Autodesk Inventor part; units mm, degrees
ref_plane "YZ Plane" through (0, 0, 0) normal (1, 0, 0) x (0, 1, 0)
ref_plane "XZ Plane" through (0, 0, 0) normal (0, 1, 0) x (-1, 0, 0)
ref_plane "XY Plane" through (0, 0, 0) normal (0, 0, 1) x (1, 0, 0)
sketch "Sketch1" plane through (0, 0, 0) normal (0, 0, 1) x (1, 0, 0)
  circle A0 centre (0, 0) radius 31.206
  dimension "d0" = 62.412
extrude "Extrusion1" add sketch "Sketch1" along normal blind 3.175
sketch "Sketch2" plane through (0, 0, 3.175) normal (0, 0, 1) x (1, 0, 0)
  circle A0 centre (0, 0) radius 31.206
  circle A1 centre (0, 0) radius 29.5
  dimension "d3" = 59
sketch "Sketch3" plane through (0, 0, 3.175) normal (0, 0, 1) x (1, 0, 0)
  line L0 (0, 0) -> (-20, 0)
  line L1 (-20, 0) -> (-20, 18)
  line L2 (-20, 18) -> (-23.175, 18)
  line L3 (-23.175, 18) -> (-23.175, -18)
  line L4 (-23.175, -18) -> (-20, -18)
  line L5 (-20, -18) -> (-20, 18)
  dimension "d4" = 20
  dimension "d5" = 18
  dimension "d6" = 3.175
  dimension "d7" = 36
extrude "Extrusion2" add sketch "Sketch3" along normal blind 52
sketch "Sketch4" plane through (-20, -18, 3.175) normal (1, 0, 0) x (0, 0, -1)
  line L0 (0, 49.206) -> (0, -13.206)
  line L1 (-52, 36) -> (-52, 0)
  line L2 (-27, 18) -> (-3, 18)
  line L3 (-3, 18) -> (-51, 18)
  line L4 (-27, 18) -> (-41, 18)
  line L5 (-41, 18) -> (-13, 18)
  circle A0 centre (-41, 18) radius 10
  circle A1 centre (-13, 18) radius 10
  line L6 (-13, 18) -> (-41, 18)
  line L7 (-41, 18) -> (-41, 24.5)
  line L8 (-41, 24.5) -> (-13, 24.5)
  line L9 (-13, 24.5) -> (-13, 18)
  line L10 (-41, 24.5) -> (-13, 24.5)
  line L11 (-13, 24.5) -> (-13, 11.5)
  line L12 (-13, 11.5) -> (-41, 11.5)
  line L13 (-41, 11.5) -> (-41, 24.5)
  point P0 (3.175, 18)
  dimension "d34" = 24
  dimension "d35" = 48
  dimension "d36" = 14
  dimension "d37" = 28
  dimension "d38" = 20
  dimension "d39" = 20
  dimension "d40" = 6.5
  dimension "d41" = 13
extrude "Extrusion3" add sketch "Sketch2" along normal blind 52
sketch "Sketch5" plane through (0, 0, 3.175) normal (0, 0, 1) x (1, 0, 0)
  line L0 (0, 0) -> (0, 23)
  line L1 (0, 23) -> (11.5, 23)
  line L2 (11.5, 23) -> (-11.5, 23)
  line L3 (-11.5, 23) -> (-11.5, -23)
  line L4 (-11.5, -23) -> (11.5, -23)
  line L5 (11.5, -23) -> (11.5, 23)
  circle A0 centre (-11.5, 23) radius 3.5
  circle A1 centre (11.5, 23) radius 3.5
  circle A2 centre (-11.5, -23) radius 3.5
  circle A3 centre (11.5, -23) radius 3.5
  dimension "d16" = 23
  dimension "d17" = 11.5
  dimension "d18" = 23
  dimension "d19" = 46
  dimension "d20" = 7
  dimension "d21" = 7
  dimension "d22" = 7
  dimension "d23" = 7
extrude "Extrusion4" add sketch "Sketch5" along normal blind 52 contours A1 L5 L1 | L1 L5 A1 | A0 L3 L2 | L2 L3 A0 | A3 L4 L5 | L5 L4 A3 | A2 L4 L3 | L3 L4 A2
sketch "Sketch6" plane through (-11.5, 23, 55.175) normal (0, 0, 1) x (1, 0, 0)
  circle A0 centre (0, 0) radius 3.5
  circle A1 centre (23, 0) radius 3.5
  circle A2 centre (23, -46) radius 3.5
  circle A3 centre (0, -46) radius 3.5
  point P0 (11.5, -23)
hole "Hole1" at (-11.5, 23, 55.175) at (11.5, 23, 55.175) at (11.5, -23, 55.175) at (-11.5, -23, 55.175) direction (0, 0, -1) diameter 3.5 depth 3.5
extrude "Extrusion5" cut sketch "Sketch4" along normal blind 52
sketch "Sketch7" plane through (0, 0, 55.175) normal (0, 0, 1) x (1, 0, 0)
  line L0 (-20, 18) -> (-23.175, 18)
  line L1 (-23.175, 18) -> (-23.175, -18)
  line L2 (-20, 18) -> (-23.175, 18)
  line L3 (-23.175, 18) -> (-23.175, -18)
  line L4 (-23.175, -18) -> (-20, -18)
  line L5 (-20, -18) -> (-20, 18)
  point P0 (0, 0)
extrude "Extrusion6" cut sketch "Sketch7" against normal blind 52
properties part number "LidarLiteV3Lid"
Source: CAD feature listing. Evaluate the final solid. Frame: model axes, mm. A direction names the side the tool comes from. Coordinates: 2 decimals unless noted, no trailing zeros. Write each loop counter-clockwise with the first axis right and the second up, starting at its lowest first coordinate (ties: lowest second). Pieces come first, ordered by that corner, then holes. Notation, with made-up numbers: (49.5, -2) -> (69.5, -2) arc R16 cw to (69.5, 9) -> close; hole circle Ø7 at (45, 84). An arc over 180 degrees is marked (long way). Return JSON: item names as keys, results as strings. Group by question number.
1) Contact query for flat-ended pins moving along their axis: P1, Ø1, axis at x = 4, y = -0.5, coming from the +Z side (3 decimals); P2, Ø1, axis at x = -11.5, y = 23, coming from the +Z side (3 decimals); P3, Ø5, axis at y = -15.5, z = 23.5, coming from the +X side. Output: stop coordinate, or through.
2) Mould query, pull axis X, two halves, no side actions, for faces 4 (the face through (-11.58, -21.25, 53.4)), 5 (the face through (30, 6.5, 30)), 6 (the face through (-24.764, 18.988, 27.201)). Classes: +X half, -X half, draft (parallel to the pull), parting line (faces both ways), or undercut.
3) Section query B-B, the plane z = 30.5. Return loops of the section in (x, y), plus the area to 3 significant figures.
4) Ray query, line 1 along X through (y, z) = (-23, 54); line 2 along Y through (x, z) = (13.5, 8); line 3 along Y through (x, z) = (9, 46.5). Return the intervals inside material, ascending.
5) Set-up query: faces 1 (the face through (29.84, 0.34, 6.18)), 2 (the face through (12, -21, 55.175)), 3 (the face through (11.42, -21.25, 53.4)). Return all of +Z, -Z, +X, -X, +Y, -Y with unobstructed straight access to the full face (end or side cutting, diameter ignored); none if empty.
6) Section query C-C, the plane x = 0. Return loops of the section in (y, z) (3 decimals), plus the area to 3 significant figures.
7) Section query A-A, the plane y = 0. Return loops of the section in (x, z) (3 decimals), plus the area to 3 significant figures.
8) Section query D-D, the plane y = 7.5. Return loops of the section in (x, z) (3 decimals).
From the geometry:
{
 "1": {"P1": "z = 3.175", "P2": "z = 51.675", "P3": "x = 28.37"},
 "2": {"face 4": "undercut", "face 5": "draft", "face 6": "parting line"},
 "3": {"outline": "circle Ø7 at (-11.5, -23); circle Ø7 at (-11.5, 23); circle Ø7 at (11.5, -23); circle Ø7 at (11.5, 23); (28.77, -6.5) arc R29.5 cw (long way) to (28.77, 6.5) -> (30.52, 6.5) arc R31.21 ccw (long way) to (30.52, -6.5) -> close", "area": "457 mm²"},
 "4": {"line 1": "-21.09 to -18.47, -15 to -13.25, -9.75 to -8, 8 to 9.75, 13.25 to 15, 18.47 to 21.09", "line 2": "-28.13 to -26.23, -25.87 to -20.13, 20.13 to 25.87, 26.23 to 28.13", "line 3": "-29.88 to -28.09, -25.45 to -20.55, 20.55 to 25.45, 28.09 to 29.88"},
 "5": {"face 1": "+X", "face 2": "+Z, +X, -X, +Y, -Y", "face 3": "+Z"},
 "6": {"outline": "(-31.206, 0) -> (31.206, 0) -> (31.206, 55.175) -> (29.5, 55.175) -> (29.5, 3.175) -> (-29.5, 3.175) -> (-29.5, 55.175) -> (-31.206, 55.175) -> close", "area": "376 mm²"},
 "7": {"outline": "(-31.206, 0) -> (31.206, 0) -> (31.206, 6.175) -> (29.5, 6.175) -> (29.5, 3.175) -> (-29.5, 3.175) -> (-29.5, 55.175) -> (-31.206, 55.175) -> close; (29.5, 54.175) -> (31.206, 54.175) -> (31.206, 55.175) -> (29.5, 55.175) -> close", "area": "294 mm²"},
 "8": {"outline": "(-30.291, 0) -> (30.291, 0) -> (30.291, 9.561) -> (28.531, 9.561) -> (28.531, 3.175) -> (-28.531, 3.175) -> (-28.531, 55.175) -> (-30.291, 55.175) -> close; (28.531, 22.789) -> (30.291, 22.789) -> (30.291, 37.561) -> (28.531, 37.561) -> close; (28.531, 50.789) -> (30.291, 50.789) -> (30.291, 55.175) -> (28.531, 55.175) -> close"}
}
